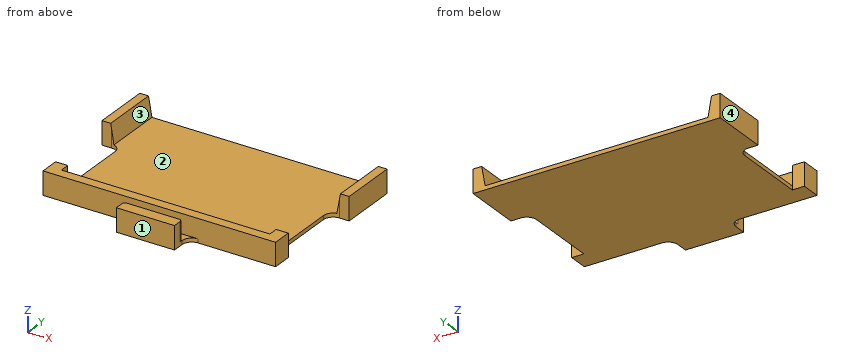
```python
from build123d import *

# Parameters (mm, degrees)
F0_W     = 6
F0_H     = 1
F0_H_2   = 1.2
F0_W_2   = 1.1
F0_H_3   = 6
F0_W_3   = 0.9
F5_DEPTH = 6
F6_R     = 1
F7_R     = 0.3


with BuildPart() as f2:
    # F2: sweep along a path in F1
    with BuildLine(Plane.XZ) as f2_path:
        Line((0, 0), (0, 0.4))
    # F0 (on Top) → F2 (sweep)
    with BuildSketch(Plane.XY):
        Polygon((-10.75, 1), (-10.75, 0), (-3, 0), (3, 0), (10.75, 0), (10.75, 1), align=None)
        Polygon((-12, 0), (-10.75, 0), (-10.75, 1), (-10.75, 2), (-12, 2), align=None)
        with Locations((0, -0.5)):
            Rectangle(F0_W, F0_H)
        Polygon((-10.75, 2), (-10.75, 1), (10.75, 1), (10.75, 2), (10.75, 10.5), (10.75, 16.5), (-10.75, 16.5), (-10.75, 10.5), align=None)
        with Locations((0, -1.6)):
            Rectangle(F0_W, F0_H_2)
        Polygon((10.75, 2), (10.75, 1), (10.75, 0), (12, 0), (12, 2), align=None)
        with Locations((-11.3, 13.5)):
            Rectangle(F0_W_2, F0_H_3)
        with Locations((-12.3, 13.5)):
            Rectangle(F0_W_3, F0_H_3)
        with Locations((11.3, 13.5)):
            Rectangle(F0_W_2, F0_H_3)
        with Locations((12.3, 13.5)):
            Rectangle(F0_W_3, F0_H_3)
    sweep(path=f2_path.line)

    # F3: sweep along a path in F1
    with BuildLine(Plane.XZ) as f3_path:
        Line((0, 0), (0, 0.4))
        Line((0, 0.4), (0, 2.4))
    # F0 (on Top) → F3 (sweep)
    with BuildSketch(Plane.XY):
        Polygon((-10.75, 1), (-10.75, 0), (-3, 0), (3, 0), (10.75, 0), (10.75, 1), align=None)
        Polygon((-12, 0), (-10.75, 0), (-10.75, 1), (-10.75, 2), (-12, 2), align=None)
        Polygon((10.75, 2), (10.75, 1), (10.75, 0), (12, 0), (12, 2), align=None)
        with Locations((12.3, 13.5)):
            Rectangle(F0_W_3, F0_H_3)
        with Locations((-12.3, 13.5)):
            Rectangle(F0_W_3, F0_H_3)
        with Locations((0, -1.6)):
            Rectangle(F0_W, F0_H_2)
    sweep(path=f3_path.line)

    # F4 (on face) → F5 (join, through all)
    with BuildSketch(Plane(origin=(0, 16.5, 0), x_dir=(-1, 0, 0), z_dir=(0, 1, 0))):
        Polygon((-11.5, 0.4), (-11.85, 2.4), (-11.85, 0.4), align=None)
        Polygon((11.85, 2.4), (11.5, 0.4), (11.85, 0.4), align=None)
    extrude(amount=-F5_DEPTH)

    # F6
    f6_edges = [f2.edges().sort_by_distance(p)[0] for p in [
        (-10.75, 10.5, 0.2),
        (10.75, 10.5, 0.2),
        (3, 0, 0.2),
        (-3, 0, 0.2),
    ]]
    fillet(f6_edges, radius=F6_R)

    # F7
    f7_edges = [f2.edges().sort_by_distance(p)[0] for p in [
        (-3, -1, 1.4),
        (3, -1, 1.4),
    ]]
    fillet(f7_edges, radius=F7_R)


solid = f2.part
```
CAD build for the part. Positions are in the model's coordinates, mm. Face numbers are marked on the shaded views. Round coordinates to 2 decimals unless told otherwise and drop trailing zeros. Loops run counter-clockwise (first coordinate to the right, second up) from the corner with the lowest first, then second, coordinate; pieces in that order, holes last. Notation, with made-up numbers: M -30,34 L -16,34 A17 ccw -16,39 Z; hole C 51.25,-11 d10. An arc over 180 degrees is marked long. Return JSON: item names as keys, results as strings. Group by question number.
(1) Saw through at B-B, the plane y = 11.75. List the corners of the cut face in (x, z), and give its area (3 significant figures).
(2) Saw through at C-C, the plane x = -1.75. List the corners of the cut face in (y, z).
(3) Mould opens along X. For the marked faces 1, 2, 3 and 4 say: +X half, -X half, draft (parallel to the pull), parting line (faces both ways), or undercut.
(4) Saw through at A-A, the plane z = 2.1. List the corners of the cut face in (x, y).
(5) Wall check: probe 1 along Y at (x, z) = (4.5, 0.7); probe 2 along Y at (x, z) = (-10, 0.3); probe 3 along Z at (x, y) = (-2.75, 8). Give the ranges that are in metal, low to high. Write a range as [from, to].
(6) Drop flat-ended pins along their axis: P1, Ø1, axis at y = 1, z = 1, coming from the +X side; P2, Ø0.6, axis at x = -11, z = 1.5, coming from the +Y side; P3, Ø3, axis at x = 3.5, y = 8, coming from the +Z side. Give the stop position or say it passes through.
(7) Saw through at D-D, the plane z = 0.7. List the corners of the cut face in (x, y), and give its area (3 significant figures).
Answer list:
{
 "1": {"outline": "M -12.75,0 L 12.75,0 L 12.75,2.4 L 11.85,2.4 L 11.5,0.4 L -11.5,0.4 L -11.85,2.4 L -12.75,2.4 Z", "area": "14.5 mm2"},
 "2": {"outline": "M -2.2,0 L 16.5,0 L 16.5,0.4 L 1,0.4 L 1,2.4 L 0,2.4 L 0,0.4 L -1,0.4 L -1,2.4 L -2.2,2.4 Z"},
 "3": {"face 1": "draft", "face 2": "undercut", "face 3": "undercut", "face 4": "-X half"},
 "4": {"outline": "M -12.75,10.5 L -11.8,10.5 L -11.8,16.5 L -12.75,16.5 Z; M -12,0 L 12,0 L 12,2 L 10.75,2 L 10.75,1 L -10.75,1 L -10.75,2 L -12,2 Z; M -3,-2.2 L 3,-2.2 L 3,-1.3 A0.3 ccw 2.7,-1 L -2.7,-1 A0.3 ccw -3,-1.3 Z; M 11.8,10.5 L 12.75,10.5 L 12.75,16.5 L 11.8,16.5 Z"},
 "5": {"probe 1": "[0, 1]", "probe 2": "[0, 16.5]", "probe 3": "[0, 0.4]"},
 "6": {"P1": "x = 12", "P2": "y = 2", "P3": "z = 0.4"},
 "7": {"outline": "M -12.75,10.5 L -11.75,10.5 A1 cw -11.55,10.48 L -11.55,16.5 L -12.75,16.5 Z; M -12,0 L 12,0 L 12,2 L 10.75,2 L 10.75,1 L -10.75,1 L -10.75,2 L -12,2 Z; M -3,-2.2 L 3,-2.2 L 3,-1.3 A0.3 ccw 2.7,-1 L -2.7,-1 A0.3 ccw -3,-1.3 Z; M 11.55,10.48 A1 cw 11.75,10.5 L 12.75,10.5 L 12.75,16.5 L 11.55,16.5 Z", "area": "48.0 mm2"}
}
